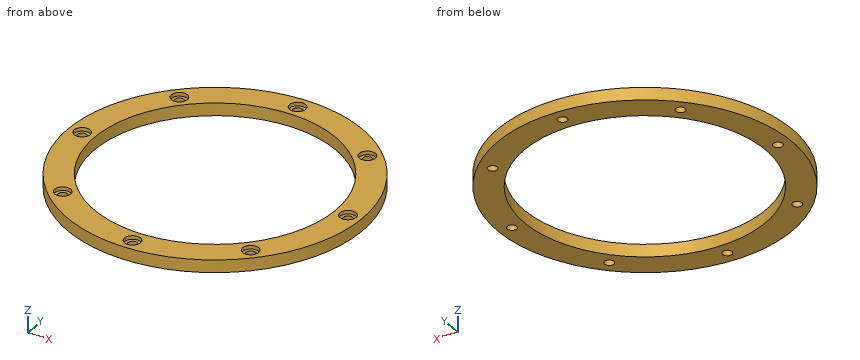
Autodesk Inventor part; units mm, degrees
ref_plane "YZ Plane" through (0, 0, 0) normal (1, 0, 0) x (0, 1, 0)
ref_plane "XZ Plane" through (0, 0, 0) normal (0, 1, 0) x (-1, 0, 0)
ref_plane "XY Plane" through (0, 0, 0) normal (0, 0, 1) x (1, 0, 0)
sketch "Skizze1" plane through (0, 0, 0) normal (0, 0, 1) x (1, 0, 0)
  circle A0 centre (0, 0) radius 67.5
  circle A1 centre (0, 0) radius 82.5
  dimension "d0" = 135
  dimension "d1" = 15
extrude "Extrusion1" add sketch "Skizze1" along normal blind 7
sketch "Skizze2" plane through (0, 0, 7) normal (0, 0, 1) x (1, 0, 0)
  circle A0 centre (0, 0) radius 67.5
  circle A1 centre (0, 0) radius 82.5
  line L0 (0, 0) -> (-82.5, 0) construction
  line L1 (-82.5, 0) -> (-67.5, 0)
  point P0 (-75, 0)
hole "Bohrung1" at (-75, 0, 7) direction (0, 0, -1) diameter 5.3 end through all counterbore diameter 9 counterbore depth 2
pattern_circular "Runde Anordnung1" count 8 over 360 about axis through (0, 0, 0) along (0, 0, 1) of "Bohrung1"
properties part number "_baseBearingMount" material "ABS-Kunststoff"
Geometry check sheet. Reference: the model listing, model coordinates, mm. Round coordinates to 2 decimals unless told otherwise and drop trailing zeros. Loops run counter-clockwise (first coordinate to the right, second up) from the corner with the lowest first, then second, coordinate; pieces in that order, holes last. Notation, with made-up numbers: (71, 39) - (80, 39) arc R26 cw to (80, 61) - close; hole circle Ø7 at (-21, 89). An arc over 180 degrees is marked (long way). Answer as CSV lines item,"result".
(1) Cross-section at B-B, the plane x = 26. Enter the section's corners in (y, z).
Output values:
outline,"(-78.3, 0) - (-62.29, 0) - (-62.29, 7) - (-78.3, 7) - close; (62.29, 0) - (78.3, 0) - (78.3, 7) - (62.29, 7) - close"
(2) Depth check by flat-ended pin: pin 1 Ø8 at (x, y) = (53.03, 53.03) entering from +Z; pin 2 Ø1 at (x, z) = (-19.5, 5.5) entering from -Y; pin 3 Ø2 at (y, z) = (-39.5, 2.5) entering from +X. Enter the tip coordinate at first touch or a pass-through.
Output values:
pin 1,"stops at z = 5"
pin 2,"stops at y = -80.28"
pin 3,"stops at x = 72.97"
(3) Material ranges on line 1 along X through (y, z) = (-51.5, 5.25); line 2 along Y through (x, z) = (55, 4.5); line 3 along X through (y, z) = (-43, 6.5), recorded low to high.
Output values:
line 1,"x = -64.45 to -57.26, -48.8 to -43.63, 43.63 to 48.8, 57.26 to 64.45"
line 2,"y = -61.49 to -54.81, -51.26 to -39.13, 39.13 to 51.26, 54.81 to 61.49"
line 3,"x = -70.41 to -52.03, 52.03 to 70.41"
(4) Cross-section at A-A, the plane x = 0. Enter the section's corners in (y, z).
Output values:
outline,"(-82.5, 0) - (-77.65, 0) - (-77.65, 5) - (-79.5, 5) - (-79.5, 7) - (-82.5, 7) - close; (-72.35, 0) - (-67.5, 0) - (-67.5, 7) - (-70.5, 7) - (-70.5, 5) - (-72.35, 5) - close; (67.5, 0) - (72.35, 0) - (72.35, 5) - (70.5, 5) - (70.5, 7) - (67.5, 7) - close; (77.65, 0) - (82.5, 0) - (82.5, 7) - (79.5, 7) - (79.5, 5) - (77.65, 5) - close"
(5) Cross-section at C-C, the plane y = 75. Enter the section's corners in (x, z), and give its area (3 significant figures).
Output values:
outline,"(-34.37, 0) - (-2.65, 0) - (-2.65, 5) - (-4.5, 5) - (-4.5, 7) - (-34.37, 7) - close; (2.65, 0) - (34.37, 0) - (34.37, 7) - (4.5, 7) - (4.5, 5) - (2.65, 5) - close"
area,"437 mm²"
